Read the model definition and answer for the solid it produces. Units are mm, in the model's axes. A direction names the side the tool comes from. Coordinates: 2 decimals unless noted, no trailing zeros. Loops run counter-clockwise (first coordinate to the right, second up) from the corner with the lowest first, then second, coordinate; pieces in that order, holes last. Notation, with made-up numbers: (75, 47.25) - (84, 47.25) arc R21 cw to (84, 77.25) - close; hole circle Ø3 at (66.25, -16.5). An arc over 180 degrees is marked (long way). Use CSV: the item, a comma, the result in double quotes.
```python
from build123d import *

# Parameters (mm, degrees)
SKETCH1_W                      = 52
SKETCH1_H                      = 32
SKETCH1_W_2                    = 11
SKETCH1_H_2                    = 23
BOSS_EXTRUDE1_DEPTH            = 11
CUT_EXTRUDE1_REACH             = 81.708
SKETCH2_R                      = 2
CUT_EXTRUDE2_REACH             = 72.426
SKETCH3_R                      = 3
CUT_EXTRUDE2_DIRECTION_2_REACH = 72.426
CUT_EXTRUDE3_REACH             = 64.04
SKETCH4_R                      = 3
CUT_EXTRUDE3_DIRECTION_2_REACH = 64.04
FILLET1_R                      = 2
FILLET2_R                      = 5.5
FILLET3_R                      = 1
SKETCH5_W                      = 13.8
SKETCH5_H                      = 6
BOSS_EXTRUDE2_DEPTH            = 11
FILLET4_R                      = 4
FILLET5_R                      = 2


with BuildPart() as part:
    # Sketch1 → Boss-Extrude1 (new body)
    # profile 1 of 2: a face of its own
    with BuildSketch(Plane(origin=(0, 0, 0), x_dir=(1, 0, 0), z_dir=(0, 1, 0))):
        with Locations((26, -16)):
            Rectangle(SKETCH1_W, SKETCH1_H)
        with Locations((26, -16.5)):
            Rectangle(SKETCH1_W_2, SKETCH1_H_2, mode=Mode.SUBTRACT)
        with Locations((11, -16.5)):
            Rectangle(SKETCH1_W_2, SKETCH1_H_2, mode=Mode.SUBTRACT)
        with Locations((41, -16.5)):
            Rectangle(SKETCH1_W_2, SKETCH1_H_2, mode=Mode.SUBTRACT)
    # profile 2 of 2: a face of its own
    with BuildSketch(Plane(origin=(0, 0, 0), x_dir=(1, 0, 0), z_dir=(0, 1, 0))):
        Polygon((15.8, -32), (7.8, -32), (7.8, -59.4), (44.2, -59.4), (44.2, -32), (36.2, -32), (36.2, -52.4), (15.8, -52.4), align=None)
    extrude(amount=BOSS_EXTRUDE1_DEPTH)

    # Sketch2 → Cut-Extrude1 (cut, up to next)
    with BuildSketch(Plane(origin=(0, 0, 0), x_dir=(-1, 0, 0), z_dir=(0, 0, -1)), mode=Mode.PRIVATE) as cut_extrude1_sk1:
        with Locations((-39, 5.5)):
            Circle(SKETCH2_R)
    cut_extrude1_tool1 = extrude(cut_extrude1_sk1.sketch, amount=-CUT_EXTRUDE1_REACH, mode=Mode.PRIVATE) & part.part
    # Sketch2 → Cut-Extrude1 (cut, up to next)
    with BuildSketch(Plane(origin=(0, 0, 0), x_dir=(-1, 0, 0), z_dir=(0, 0, -1)), mode=Mode.PRIVATE) as cut_extrude1_sk2:
        with Locations((-13, 5.5)):
            Circle(SKETCH2_R)
    cut_extrude1_tool2 = extrude(cut_extrude1_sk2.sketch, amount=-CUT_EXTRUDE1_REACH, mode=Mode.PRIVATE) & part.part
    add(cut_extrude1_tool1.solids().sort_by_distance((39, 5.5, 0))[0], mode=Mode.SUBTRACT)
    add(cut_extrude1_tool2.solids().sort_by_distance((13, 5.5, 0))[0], mode=Mode.SUBTRACT)

    # Sketch3 → Cut-Extrude2 (cut, up to next)
    with BuildSketch(Plane(origin=(15.8, 0, 0), x_dir=(0, 0, -1), z_dir=(1, 0, 0)), mode=Mode.PRIVATE) as cut_extrude2_sk1:
        with Locations((-42.2, 5.5)):
            Circle(SKETCH3_R)
    cut_extrude2_tool1 = extrude(cut_extrude2_sk1.sketch, amount=-CUT_EXTRUDE2_REACH, mode=Mode.PRIVATE) & part.part
    add(cut_extrude2_tool1.solids().sort_by_distance((15.8, 5.5, 42.2))[0], mode=Mode.SUBTRACT)

    # Sketch3 → Cut-Extrude2 direction 2 (cut, up to next)
    with BuildSketch(Plane(origin=(15.8, 0, 0), x_dir=(0, 0, -1), z_dir=(1, 0, 0)), mode=Mode.PRIVATE) as cut_extrude2_direction_2_sk1:
        with Locations((-42.2, 5.5)):
            Circle(SKETCH3_R)
    cut_extrude2_direction_2_tool1 = extrude(cut_extrude2_direction_2_sk1.sketch, amount=CUT_EXTRUDE2_DIRECTION_2_REACH, mode=Mode.PRIVATE) & part.part
    add(cut_extrude2_direction_2_tool1.solids().sort_by_distance((15.8, 5.5, 42.2))[0], mode=Mode.SUBTRACT)

    # Sketch4 → Cut-Extrude3 (cut, up to next)
    with BuildSketch(Plane.XY.offset(32), mode=Mode.PRIVATE) as cut_extrude3_sk1:
        with Locations(Location((26, 5.5, 0), (0, 0, 180))):
            Circle(SKETCH4_R)
    cut_extrude3_tool1 = extrude(cut_extrude3_sk1.sketch, amount=-CUT_EXTRUDE3_REACH, mode=Mode.PRIVATE) & part.part
    add(cut_extrude3_tool1.solids().sort_by_distance((26, 5.5, 32))[0], mode=Mode.SUBTRACT)

    # Sketch4 → Cut-Extrude3 direction 2 (cut, up to next)
    with BuildSketch(Plane.XY.offset(32), mode=Mode.PRIVATE) as cut_extrude3_direction_2_sk1:
        with Locations(Location((26, 5.5, 0), (0, 0, 180))):
            Circle(SKETCH4_R)
    cut_extrude3_direction_2_tool1 = extrude(cut_extrude3_direction_2_sk1.sketch, amount=CUT_EXTRUDE3_DIRECTION_2_REACH, mode=Mode.PRIVATE) & part.part
    add(cut_extrude3_direction_2_tool1.solids().sort_by_distance((26, 5.5, 32))[0], mode=Mode.SUBTRACT)

    # Fillet1
    fillet1_edges = [part.edges().sort_by_distance(p)[0] for p in [
        (35.5, 5.5, 28),
        (46.5, 5.5, 28),
        (46.5, 5.5, 5),
        (5.5, 5.5, 5),
        (5.5, 5.5, 28),
        (16.5, 5.5, 28),
        (20.5, 5.5, 5),
        (31.5, 5.5, 5),
        (52, 5.5, 32),
        (0, 5.5, 32),
        (0, 5.5, 0),
        (52, 5.5, 0),
    ]]
    fillet(fillet1_edges, radius=FILLET1_R)

    # Fillet2
    fillet2_edges = [part.edges().sort_by_distance(p)[0] for p in [
        (44.2, 5.5, 32),
        (7.8, 5.5, 32),
    ]]
    fillet(fillet2_edges, radius=FILLET2_R)

    # Fillet3
    fillet3_edges = [part.edges().sort_by_distance(p)[0] for p in [
        (26, 0, 52.4),
        (36.2, 0, 42.2),
        (26, 0, 32),
        (15.8, 0, 42.2),
    ]]
    fillet(fillet3_edges, radius=FILLET3_R)

    # Sketch5 → Boss-Extrude2 (add)
    with BuildSketch(Plane.XZ):
        with Locations((0.9, 56.4)):
            Rectangle(SKETCH5_W, SKETCH5_H)
        with Locations((51.1, 56.4)):
            Rectangle(SKETCH5_W, SKETCH5_H)
    extrude(amount=-BOSS_EXTRUDE2_DEPTH)

    # Fillet4
    fillet4_edges = [part.edges().sort_by_distance(p)[0] for p in [
        (7.8, 5.5, 53.4),
        (44.2, 5.5, 53.4),
    ]]
    fillet(fillet4_edges, radius=FILLET4_R)

    # Fillet5
    fillet5_edges = [part.edges().sort_by_distance(p)[0] for p in [
        (-6, 5.5, 53.4),
        (-6, 5.5, 59.4),
        (58, 5.5, 59.4),
        (58, 5.5, 53.4),
    ]]
    fillet(fillet5_edges, radius=FILLET5_R)


solid = part.part
```
Q1. Given P1, Ø2, axis at y = 8.5, z = 48.5, coming from the -X side; P2, Ø1, axis at y = 9, z = 17, coming from the +X side; P3, Ø5, axis at y = 8.5, z = 27, coming from the -X side, each flat-ended and moving along its own axis, determine where each tip first touches the part or whether it passes through.
Reported:
P1,"stops at x = 7.8"
P2,"stops at x = 52"
P3,"stops at x = 0"
Q2. For a pull along X with two mould halves and no side action, classify faces 4 (the face through (0.57, 5.58, 31.4)), 5 (the face through (40.14, 6.4, 39.34)), 6 (the face through (52, 5, 16)), 7 (the face through (28.21, 3.47, 30.03)) as +X half, -X half, draft (parallel to the pull), parting line (faces both ways), or undercut.
Reported:
face 4,"-X half"
face 5,"draft"
face 6,"+X half"
face 7,"undercut"
Q3. The part is cut by section B-B on z = 46. Determine the outline of the cut face in (x, y), and give its area (3 significant figures).
Reported:
outline,"(7.8, 0) - (14.8, 0) arc R1 ccw to (15.8, 1) - (15.8, 11) - (7.8, 11) - close; (36.2, 1) arc R1 ccw to (37.2, 0) - (44.2, 0) - (44.2, 11) - (36.2, 11) - close"
area,"176 mm²"
Q4. The part is cut by section D-D on z = 14.5. Determine the outline of the cut face in (x, y), and give its area (3 significant figures).
Reported:
outline,"(0, 0) - (5.5, 0) - (5.5, 11) - (0, 11) - close; (16.5, 0) - (20.5, 0) - (20.5, 11) - (16.5, 11) - close; (31.5, 0) - (35.5, 0) - (35.5, 11) - (31.5, 11) - close; (46.5, 0) - (52, 0) - (52, 11) - (46.5, 11) - close"
area,"209 mm²"
Q5. Find the intervals of material crossed by probe 1 along X at (y, z) = (6, 12.5); probe 2 along Y at (x, z) = (42, 42); probe 3 along Y at (x, z) = (39, 2.45), in increasing order. Write a range as [from, to].
Reported:
probe 1,"x = [0, 5.5], [16.5, 20.5], [31.5, 35.5], [46.5, 52]"
probe 2,"y = [0, 2.51], [8.49, 11]"
probe 3,"y = [0, 3.5], [7.5, 11]"
Q6. A tool of negligible diameter and unlimited length cuts with its end or side. For faces 1 (the face through (51.43, 5.58, 31.4)), 2 (the face through (24, 8, 32)), 3 (the face through (57.4, 5.58, 58.83)), from which of +Z, -Z, +X, -X, +Y, -Y can it reach the whole face along a straight path? Write none if from no direction.
Reported:
face 1,"+X, +Y, -Y"
face 2,"+Y, -Y"
face 3,"+Z, +X, +Y, -Y"
Q7. The part is cut by section C-C on x = 9. Determine the outline of the cut face in (y, z).
Reported:
outline,"(0, 0) - (11, 0) - (11, 5) - (0, 5) - close; (0, 28) - (11, 28) - (11, 59.4) - (0, 59.4) - close; hole circle Ø6 at (5.5, 42.2)"
Q8. The part is cut by section A-A on x = 39. Determine the outline of the cut face in (y, z), and give its area (3 significant figures).
Reported:
outline,"(0, 0) - (3.5, 0) - (3.5, 5) - (0, 5) - close; (0, 28) - (11, 28) - (11, 59.4) - (0, 59.4) - close; (7.5, 0) - (11, 0) - (11, 5) - (7.5, 5) - close; hole circle Ø6 at (5.5, 42.2)"
area,"352 mm²"
